```python
from build123d import *

# Parameters (mm, degrees)
F0_R     = 26
F0_R_2   = 24.5
F1_DEPTH = 55
F2_R     = 24.5
F2_R_2   = 21.5
F3_DEPTH = 21.5
F4_SIZE  = 2
F5_SIZE  = 1


with BuildPart() as f1:
    # F0 (on Front) → F1 (new body)
    with BuildSketch(Plane.XZ):
        Circle(F0_R)
        Circle(F0_R_2, mode=Mode.SUBTRACT)
    extrude(amount=F1_DEPTH)

    # F2 (on face) → F3 (join)
    with BuildSketch(Plane.XZ.offset(55)):
        Circle(F2_R)
        Circle(F2_R_2, mode=Mode.SUBTRACT)
    extrude(amount=-F3_DEPTH)

    # F4
    f4_edges = [f1.edges().sort_by_distance(p)[0] for p in [
        (-26, -55, 0),
    ]]
    chamfer(f4_edges, length=F4_SIZE)

    # F5
    f5_edges = [f1.edges().sort_by_distance(p)[0] for p in [
        (-24.5, 0, 0),
    ]]
    chamfer(f5_edges, length=F5_SIZE)


solid = f1.part
```
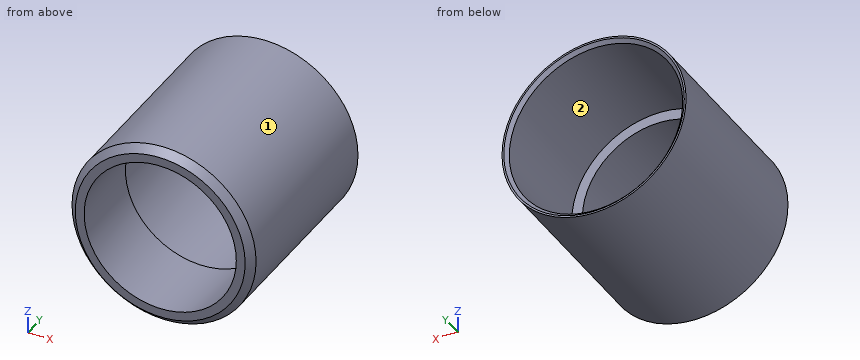
Could you check a few things on this model? Use its own coordinates, in mm. Face numbers are marked on the shaded views. Round coordinates to 2 decimals unless told otherwise and drop trailing zeros. Order: outer loops, then holes, each group sorted by start corner. A loop starts at its lowest first (then second) coordinate and runs counter-clockwise, first axis right, second up. Notation, with made-up numbers: M 85.25,88.25 L 143.25,88.25 A13 ccw 143.25,92.25 Z; hole C 86.25,76 d7. An arc over 180 degrees is marked long. One line per question, with ' | ' between items. Start each with the question number.
(1) Suppose I cut it at A-A on x = 0. List the corners of the cut face in (y, z) for me, then the cut area to 3 significant figures.
(2) Suppose I cut it at D-D on y = -24. List the corners of the cut face in (x, z) for me.
(3) Suppose I cut it at B-B on z = 0. List the corners of the cut face in (x, y) for me, then the cut area to 3 significant figures.
(4) Suppose I cut it at C-C on y = -51. List the corners of the cut face in (x, z) for me, then the cut area to 3 significant figures.
(5) Please list where these lines run through material, in increasing order: line 1 along X through (y, z) = (-17.5, -5); line 2 along Z through (x, y) = (0, -17); line 3 along Z through (x, y) = (0, -38.75).
(6) For P1, Ø1, axis at x = 6, y = -22.5, coming from the -Z side; P2, Ø10, axis at x = 14.5, y = -19, coming from the +Z side; P3, Ø5, axis at x = -11, z = -17, coming from the -Y side; P4, Ø2, axis at y = -49, z = 10, coming from the +X side, each with a flat end and sliding along its axis, tell me the tip position at first contact or that it passes through.
(7) Thinking about a two-plate mould opening in X: for the marked faces 1 and 2, which applies, +X half, -X half, draft (parallel to the pull), parting line (faces both ways), or undercut?
Geometry results:
1) outline: M -55,-24 L -53,-26 L 0,-26 L 0,-25.5 L -1,-24.5 L -33.5,-24.5 L -33.5,-21.5 L -55,-21.5 Z; M -55,21.5 L -33.5,21.5 L -33.5,24.5 L -1,24.5 L 0,25.5 L 0,26 L -53,26 L -55,24 Z | area: 289 mm²
2) outline: C 0,0 d52; hole C 0,0 d49
3) outline: M -26,-53 L -24,-55 L -21.5,-55 L -21.5,-33.5 L -24.5,-33.5 L -24.5,-1 L -25.5,0 L -26,0 Z; M 21.5,-55 L 24,-55 L 26,-53 L 26,0 L 25.5,0 L 24.5,-1 L 24.5,-33.5 L 21.5,-33.5 Z | area: 289 mm²
4) outline: C 0,0 d52; hole C 0,0 d43 | area: 672 mm²
5) line 1: -25.51 to -23.98, 23.98 to 25.51 | line 2: -26 to -24.5, 24.5 to 26 | line 3: -26 to -21.5, 21.5 to 26
6) P1: z = -25.41 | P2: z = 24.2 | P3: y = -55 | P4: x = 24.39
7) face 1: parting line | face 2: undercut
